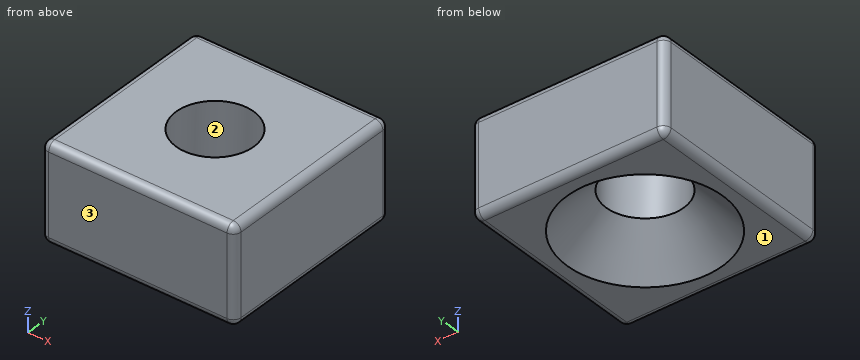
from build123d import *

# Parameters (mm, degrees)
F0_W     = 12.7
F0_H     = 12.7
F0_R     = 2.54
F1_DEPTH = 6.35
F2_SIZE  = 2.54
F3_R     = 0.508


with BuildPart() as f1:
    # F0 (on Top) → F1 (new body)
    with BuildSketch(Plane.XY):
        Rectangle(F0_W, F0_H)
        Circle(F0_R, mode=Mode.SUBTRACT)
    extrude(amount=F1_DEPTH)

    # F2
    f2_edges = [f1.edges().sort_by_distance(p)[0] for p in [
        (-2.54, 0, 0),
    ]]
    chamfer(f2_edges, length=F2_SIZE)

    # F3
    f3_edges = [f1.edges().sort_by_distance(p)[0] for p in [
        (0, -6.35, 0),
        (6.35, 0, 0),
        (0, 6.35, 0),
        (-6.35, 0, 0),
        (-6.35, -6.35, 3.175),
        (6.35, -6.35, 3.175),
        (6.35, 6.35, 3.175),
        (-6.35, 6.35, 3.175),
        (0, 6.35, 6.35),
        (-6.35, 0, 6.35),
        (0, -6.35, 6.35),
        (6.35, 0, 6.35),
    ]]
    fillet(f3_edges, radius=F3_R)


solid = f1.part
Model file for the job. Use its own axes, mm. Face numbers are marked on the shaded views. Give positions to 0.01 mm unless a question says otherwise; leave off trailing zeros. Order: outer loops, then holes, each group sorted by start corner. A loop starts at its lowest first (then second) coordinate and runs counter-clockwise, first axis right, second up. Notation, with made-up numbers: M 27.25,51 L 78.25,51 A20 ccw 78.25,81 Z; hole C -14.75,57 d3. An arc over 180 degrees is marked long. Write item = value, one per line.
Q1. Drill centre lines: line 1 (Y direction, x = 0, z = 3.75); line 2 (Y direction, x = 2, z = 4.5); line 3 (X direction, y = -0.5, z = 4.75). Where is each one in solid material? Low to high. Write a range as [from, to].
Derived:
line_1 = [-6.35, -2.54], [2.54, 6.35]
line_2 = [-6.35, -1.57], [1.57, 6.35]
line_3 = [-6.35, -2.49], [2.49, 6.35]
Q2. Cut at C-C, the plane z = 4.75. List the corners of the cut face in (x, y).
Derived:
outline = M -6.35,-5.84 A0.51 ccw -5.84,-6.35 L 5.84,-6.35 A0.51 ccw 6.35,-5.84 L 6.35,5.84 A0.51 ccw 5.84,6.35 L -5.84,6.35 A0.51 ccw -6.35,5.84 Z; hole C 0,0 d5.08
Q3. Cut at A-A, the plane y = 0. List the corners of the cut face in (x, z).
Derived:
outline = M -6.35,0.51 A0.51 ccw -5.84,0 L -5.08,0 L -2.54,2.54 L -2.54,6.35 L -5.84,6.35 A0.51 ccw -6.35,5.84 Z; M 2.54,2.54 L 5.08,0 L 5.84,0 A0.51 ccw 6.35,0.51 L 6.35,5.84 A0.51 ccw 5.84,6.35 L 2.54,6.35 Z
Q4. Two-plate mould, pull along Y, no slides. Class the marked faces 1, 2 and 3: pulls with the +Y half, pulls with the -Y half, needs draft (parallel to the pull), parting line crosses it, or undercut.
Derived:
face_1 = needs draft
face_2 = undercut
face_3 = pulls with the -Y half
Q5. Flat gauge pin, fed straight in: pin 1 (6 mm diameter, centred on x = -1.5, y = -3.5, fed in from -Z). Where does the tip first touch, or does it go through?
Derived:
pin_1 = 0
